Answer from the drawing. Dimensions are ordinates in mm from the lowest x, y and z of the part. A direction names the side the tool comes from. Coordinates: 2 decimals unless noted, no trailing zeros. Loops run counter-clockwise (first coordinate to the right, second up) from the corner with the lowest first, then second, coordinate; pieces in that order, holes last. Notation, with made-up numbers: M 13.25,10.25 L 47.25,10.25 A10 ccw 47.25,18.25 Z; hole C 84,23.25 d4. An arc over 180 degrees is marked long. One line per item, written item: value. Start each with the question number.
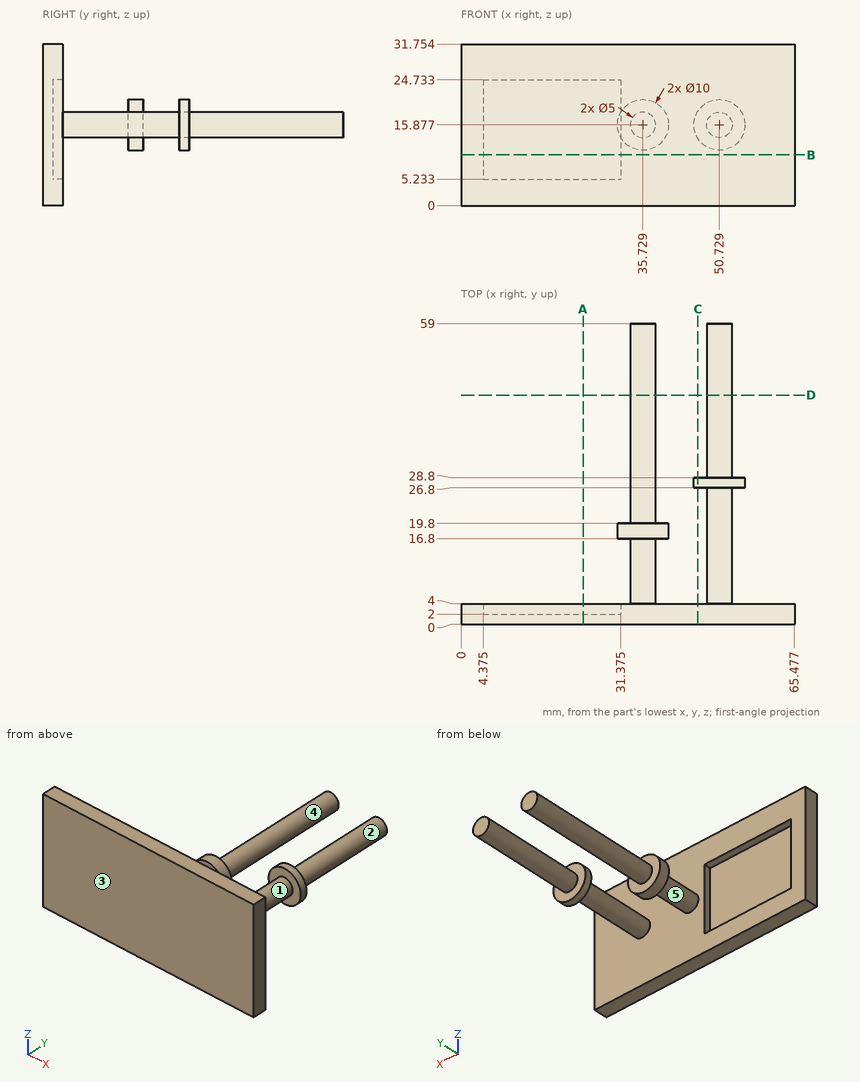
1) Section A-A (x = 24) is taken. Determine the outline of the cut face in (y, z).
2) For a pull along Y with two mould halves and no side action, classify the marked faces 3, 4 and 5 as released by +Y, released by -Y, zero draft, split by the parting line, or undercut.
3) A tool of negligible diameter and unlimited length cuts with its end or side. For the marked faces 1 and 2, from which of +Z, -Z, +X, -X, +Y, -Y can it reach the whole face along a straight path? Write none if from no direction.
4) Section D-D (y = 45) is taken. Determine the outline of the cut face in (x, z).
5) Consider line 1 along Y through (x, z) = (49, 12.5); line 2 along Z through (x, y) = (36, 21); line 3 along Y through (x, z) = (38, 7.5). Determine where each line is inside the solid, lowest interval first.
6) Section B-B (z = 10) is taken. Determine the outline of the cut face in (x, y) (1 decimal), then the cut area to 3 significant figures.
7) Section C-C (x = 46.5) is taken. Determine the outline of the cut face in (y, z) (1 decimal).
8) Flat-ended cylindrical pins translate along their axes: pin 1 (10 mm diameter, centred on x = 16.5, z = 17.5, fed in from +Y); pin 2 (12 mm diameter, centred on x = 26.5, z = 23, fed in from +Y); pin 3 (6 mm diameter, centred on x = 41, y = 10, fed in from +Z) (1 decimal). Find the tip coordinate at first contact, or state that the pin passes through.
Results found:
1. outline: M 0,0 L 4,0 L 4,5.23 L 2,5.23 L 2,24.73 L 4,24.73 L 4,31.75 L 0,31.75 Z
2. face 3: released by -Y
2. face 4: zero draft
2. face 5: undercut
3. face 1: none
3. face 2: +Y
4. outline: C 35.73,15.88 d5; C 50.73,15.88 d5
5. line 1: y = 0 to 4, 26.8 to 28.8
5. line 2: z = 13.39 to 18.36
5. line 3: y = 0 to 4
6. outline: M 0,0 L 65.5,0 L 65.5,4 L 31.4,4 L 31.4,2 L 4.4,2 L 4.4,4 L 0,4 Z
6. area: 208 mm²
7. outline: M 0,0 L 4,0 L 4,31.8 L 0,31.8 Z; M 26.8,13.2 L 28.8,13.2 L 28.8,18.5 L 26.8,18.5 Z
8. pin 1: stops at y = 2
8. pin 2: stops at y = 4
8. pin 3: stops at z = 16.9
